from build123d import *

# Parameters (mm, degrees)
SKETCH_2_W           = 65.2997206
SKETCH_2_H           = 38
SKETCH_2_R           = 1.00000254
SKETCH_2_R_2         = 0.922218434
SKETCH_2_R_3         = 1.5
EXTRUDE_2_DEPTH      = 4.5
SKETCH_3_R           = 1.5
CUT_EXTRUDE_2_DEPTH  = 2.5
SKETCH_5_W           = 65.2997206
SKETCH_5_H           = 38
SKETCH_5_W_2         = 61.2997206
SKETCH_5_H_2         = 34
EXTRUDE_3_DEPTH      = 21
EXTRUDE_3_DEPTH_BACK = 16
SKETCH_7_W           = 8.214112973
SKETCH_7_H           = 3.795011114
CUT_EXTRUDE_4_DEPTH  = 3
SKETCH_8_W           = 4
SKETCH_8_H           = 9.575559499
CUT_EXTRUDE_5_DEPTH  = 3
SKETCH_9_W           = 9.326303795
SKETCH_9_H           = 4.202278939
CUT_EXTRUDE_6_DEPTH  = 3
CUT_EXTRUDE_7_DEPTH  = 10
SKETCH_15_R          = 1.75
CUT_EXTRUDE_8_DEPTH  = 1.5
SKETCH_18_W          = 61.2997206
SKETCH_18_H          = 35
CUT_EXTRUDE_9_DEPTH  = 2
SKETCH_19_W          = 2
SKETCH_19_H          = 4
CUT_EXTRUDE_10_DEPTH = 2
SKETCH_20_W          = 2
SKETCH_20_H          = 8
CUT_EXTRUDE_11_DEPTH = 1.2
SKETCH_21_W          = 2
SKETCH_21_H          = 8
CUT_EXTRUDE_12_DEPTH = 2


with BuildPart() as part:
    # 草图2 → 凸台-拉伸2 (new body)
    with BuildSketch(Plane(origin=(0, 0, -6), x_dir=(-1, 0, 0), z_dir=(0, 0, -1))):
        with Locations((29.273558547, -24.066548133)):
            Rectangle(SKETCH_2_W, SKETCH_2_H)
        with Locations((1.016002032, -11.24978156)):
            Circle(SKETCH_2_R, mode=Mode.SUBTRACT)
        with Locations((0.889001778, -36.83007366)):
            Circle(SKETCH_2_R, mode=Mode.SUBTRACT)
        with Locations((57.658115316, -36.64983236)):
            Circle(SKETCH_2_R, mode=Mode.SUBTRACT)
        with Locations((57.658115316, -11.24978156)):
            Circle(SKETCH_2_R_2, mode=Mode.SUBTRACT)
        with Locations((29.273558547, -32.316548133)):
            Circle(SKETCH_2_R_3, mode=Mode.SUBTRACT)
        with BuildLine():
            Line((27.785407033, -15.816548133), (27.785407033, -13.183619987))
            ThreePointArc((27.785407033, -13.183619987), (29.273558547, -11.695468472), (30.761710061, -13.183619987))
            Line((30.761710061, -13.183619987), (30.761710061, -15.816548133))
            ThreePointArc((30.761710061, -15.816548133), (29.273558547, -17.304699647), (27.785407033, -15.816548133))
        make_face(mode=Mode.SUBTRACT)
    extrude(amount=EXTRUDE_2_DEPTH)

    # 草图3 → 切除-拉伸2 (cut)
    with BuildSketch(Plane(origin=(0, 0, -6), x_dir=(-1, 0, 0), z_dir=(0, 0, -1))):
        Polygon((29.273558547, -18.991974614), (32.023558547, -17.404261373), (32.023558547, -14.920341582), (32.023558547, -14.228834893), (32.023558547, -11.744915102), (29.273558547, -10.157201862), (26.523558547, -11.744915102), (26.523558547, -14.228834893), (26.523558547, -14.920341582), (26.523558547, -17.404261373), align=None)
        with BuildLine():
            ThreePointArc((30.761710061, -15.816548133), (29.273558547, -17.304699647), (27.785407033, -15.816548133))
            Line((27.785407033, -15.816548133), (27.785407033, -13.183619987))
            ThreePointArc((27.785407033, -13.183619987), (29.273558547, -11.695468472), (30.761710061, -13.183619987))
            Line((30.761710061, -13.183619987), (30.761710061, -15.816548133))
        make_face(mode=Mode.SUBTRACT)
        Polygon((26.523558547, -30.728834893), (26.523558547, -33.904261373), (29.273558547, -35.491974614), (32.023558547, -33.904261373), (32.023558547, -30.728834893), (29.273558547, -29.141121653), align=None)
        with Locations((29.273558547, -32.316548133)):
            Circle(SKETCH_3_R, mode=Mode.SUBTRACT)
    extrude(amount=CUT_EXTRUDE_2_DEPTH, mode=Mode.SUBTRACT)

    # 草图5 → 凸台-拉伸3 (add, two sides)
    with BuildSketch(Plane(origin=(0, 0, -10.5), x_dir=(-1, 0, 0), z_dir=(0, 0, -1))) as extrude_3_sk:
        with Locations((29.273558547, -24.066548133)):
            Rectangle(SKETCH_5_W, SKETCH_5_H)
        with Locations((29.273558547, -24.066548133)):
            Rectangle(SKETCH_5_W_2, SKETCH_5_H_2, mode=Mode.SUBTRACT)
    extrude(amount=EXTRUDE_3_DEPTH)
    extrude(extrude_3_sk.sketch, amount=-EXTRUDE_3_DEPTH_BACK)

    # 草图7 → 切除-拉伸4 (cut)
    with BuildSketch(Plane(origin=(0, -5.066548133, 0), x_dir=(1, 0, 0), z_dir=(0, 1, 0))):
        with Locations((-50.955145133, -3.662545243)):
            Rectangle(SKETCH_7_W, SKETCH_7_H)
    extrude(amount=-CUT_EXTRUDE_4_DEPTH, mode=Mode.SUBTRACT)

    # 草图8 → 切除-拉伸5 (cut)
    with BuildSketch(Plane.ZY.offset(61.923418847)):
        with Locations((3.6000508, -23.483057223)):
            Rectangle(SKETCH_8_W, SKETCH_8_H)
    extrude(amount=-CUT_EXTRUDE_5_DEPTH, mode=Mode.SUBTRACT)

    # 草图9 → 切除-拉伸6 (cut)
    with BuildSketch(Plane.XZ.offset(43.066548133)):
        with Locations((-44.464129124, 3.49891133)):
            Rectangle(SKETCH_9_W, SKETCH_9_H)
    extrude(amount=-CUT_EXTRUDE_6_DEPTH, mode=Mode.SUBTRACT)

    # 草图13 → 切除-拉伸7 (cut)
    with BuildSketch(Plane.XY.offset(-6)):
        Polygon((-59.923418847, -16.066514367), (-59.923418847, -19.252115931), (-54.525349934, -19.252115931), (-54.525349934, -41.066548133), (-34.525349934, -41.066548133), (-34.525349934, -7.066548133), (-54.525349934, -7.066548133), (-54.525349934, -12.880912803), (-54.525349934, -16.066514367), align=None)
    extrude(amount=-CUT_EXTRUDE_7_DEPTH, mode=Mode.SUBTRACT)

    # 草图15 → 切除-拉伸8 (cut)
    with BuildSketch(Plane(origin=(0, 0, -10.5), x_dir=(-1, 0, 0), z_dir=(0, 0, -1))):
        with Locations((1.016002032, -11.24978156)):
            Circle(SKETCH_15_R)
        with Locations((57.658115316, -11.24978156)):
            Circle(SKETCH_15_R)
        with Locations((0.889001778, -36.83007366)):
            Circle(SKETCH_15_R)
        with Locations((57.658115316, -36.64983236)):
            Circle(SKETCH_15_R)
    extrude(amount=-CUT_EXTRUDE_8_DEPTH, mode=Mode.SUBTRACT)

    # 草图18 → 切除-拉伸9 (cut)
    with BuildSketch(Plane(origin=(0, 0, -31.5), x_dir=(-1, 0, 0), z_dir=(0, 0, -1))):
        with Locations((29.273558547, -24.066548133)):
            Rectangle(SKETCH_18_W, SKETCH_18_H)
    extrude(amount=-CUT_EXTRUDE_9_DEPTH, mode=Mode.SUBTRACT)

    # 草图19 → 切除-拉伸10 (cut)
    with BuildSketch(Plane.ZY.offset(-1.376301753)):
        with Locations((-28.5, -9.066548133)):
            Rectangle(SKETCH_19_W, SKETCH_19_H)
        with Locations((-28.5, -39.066548133)):
            Rectangle(SKETCH_19_W, SKETCH_19_H)
    extrude(amount=-CUT_EXTRUDE_10_DEPTH, mode=Mode.SUBTRACT)

    # 草图20 → 切除-拉伸11 (cut)
    with BuildSketch(Plane(origin=(0, 0, -31.5), x_dir=(-1, 0, 0), z_dir=(0, 0, -1))):
        with Locations((60.923418847, -24.066548133)):
            Rectangle(SKETCH_20_W, SKETCH_20_H)
    extrude(amount=-CUT_EXTRUDE_11_DEPTH, mode=Mode.SUBTRACT)

    # 草图21 → 切除-拉伸12 (cut)
    with BuildSketch(Plane.ZY.offset(61.923418847)):
        with Locations((-27.7, -24.066548133)):
            Rectangle(SKETCH_21_W, SKETCH_21_H)
    extrude(amount=-CUT_EXTRUDE_12_DEPTH, mode=Mode.SUBTRACT)


solid = part.part
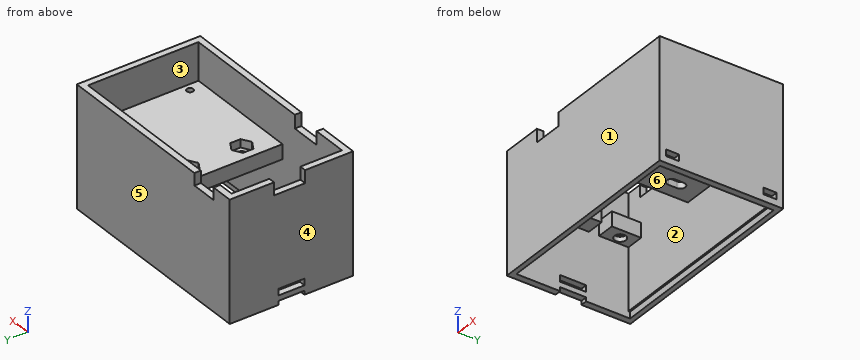
CAD build for the part. Positions are in the model's coordinates, mm. Face numbers are marked on the shaded views. A direction names the side the tool comes from. Round coordinates to 2 decimals unless told otherwise and drop trailing zeros. Order: outer loops, then holes, each group sorted by start corner. A loop starts at its lowest first (then second) coordinate and runs counter-clockwise, first axis right, second up. Notation, with made-up numbers: (-26.5, -10) -> (-5.5, -10) arc R28 cw to (-5.5, 18) -> close; hole circle Ø10 at (35.5, 3.25). An arc over 180 degrees is marked (long way). Write item = value, one per line. Start each with the question number.
(1) Pin check, flat tips, straight feed: P1, Ø1, axis at x = -61, y = -26, coming from the +Z side; P2, Ø10, axis at x = -11, y = -25, coming from the -Z side; P3, Ø5, axis at x = -14, y = -20.5, coming from the +Z side. Stop position of each tip, or through.
(2) Cut at C-C, the plane x = -45.5. List the corners of the cut face in (y, z).
(3) Cut at B-B, the plane y = -26. List the corners of the cut face in (x, z).
(4) Pull direction X, two halves, no side cores. Call the marked faces 4, 5 and 6: released by +X, released by -X, zero draft, split by the parting line, or undercut.
(5) Cut at D-D, the plane x = -24. List the corners of the cut face in (y, z), then the cut area to 3 significant figures.
(6) Which spindle directions (+Z, -Z, +X, -X, +Y, -Y) get a long thin tool onto all of the face, cutting with end or side? Do the marked faces 1, 2 and 3. Say none if no direction does.
(7) Probe line 1 (X direction, y = -34.5, z = -18.5); line 2 (Y direction, x = -40, z = -5); line 3 (X direction, y = -21, z = -27). List the from-to ranges inside material, lowest first. Write a range as [from, to].
(8) Cut at A-A, the plane z = -17.5. List the corners of the cut face in (x, y), then the cut area to 3 significant figures.
Model answer:
q1.P1 = 1.6
q1.P2 = -10.5
q1.P3 = -6
q2.outline = (-43.07, -31.5) -> (-41.57, -31.5) -> (-41.57, -29.5) -> (-41.07, -29.5) -> (-41.07, 1.4) -> (-43.07, 1.4) -> close; (-7.07, -29.5) -> (-6.57, -29.5) -> (-6.57, -31.5) -> (-5.07, -31.5) -> (-5.07, 5.5) -> (-7.07, 5.5) -> close
q3.outline = (-61.92, -30.3) -> (-59.92, -30.3) -> (-59.92, -28.7) -> (-61.92, -28.7) -> close; (-61.92, -26.7) -> (-59.92, -26.7) -> (-59.92, -10.5) -> (-54.53, -10.5) -> (-54.53, -6) -> (-59.92, -6) -> (-59.92, 1.6) -> (-61.92, 1.6) -> close; (-34.53, -10.5) -> (1.38, -10.5) -> (1.38, -31.5) -> (3.38, -31.5) -> (3.38, 5.5) -> (1.38, 5.5) -> (1.38, -6) -> (-34.53, -6) -> close
q4.face_4 = released by -X
q4.face_5 = zero draft
q4.face_6 = undercut
q5.outline = (-43.07, -31.5) -> (-41.57, -31.5) -> (-41.57, -29.5) -> (-41.07, -29.5) -> (-41.07, -10.5) -> (-7.07, -10.5) -> (-7.07, -29.5) -> (-6.57, -29.5) -> (-6.57, -31.5) -> (-5.07, -31.5) -> (-5.07, 5.5) -> (-7.07, 5.5) -> (-7.07, -6) -> (-41.07, -6) -> (-41.07, 5.5) -> (-43.07, 5.5) -> close
q5.area = 299 mm2
q6.face_1 = +Z, -Z, +X, -X, -Y
q6.face_2 = none
q6.face_3 = +Z
q7.line_1 = [-61.92, -59.92], [1.38, 3.38]
q7.line_2 = [-43.07, -41.07], [-7.07, -5.07]
q7.line_3 = [1.38, 3.38]
q8.outline = (-61.92, -43.07) -> (3.38, -43.07) -> (3.38, -5.07) -> (-61.92, -5.07) -> close; hole (-59.92, -41.07) -> (1.38, -41.07) -> (1.38, -7.07) -> (-59.92, -7.07) -> close
q8.area = 397 mm2
